from build123d import *

# Parameters (mm, degrees)
F0_W      = 16.5
F0_H      = 32.5
F1_DEPTH  = 14
F3_W      = 16.5
F3_H      = 17
F4_DEPTH  = 10
F5_W      = 4
F5_H      = 17
F6_DEPTH  = 14.001
F7_W      = 8.5
F7_H      = 4.5
F8_DEPTH  = 14.001
F9_R      = 2.85
F10_DEPTH = 3
F11_R     = 1
F12_DEPTH = 10


with BuildPart() as f1:
    # F0 (on Top) → F1 (new body)
    with BuildSketch(Plane.XY):
        Rectangle(F0_W, F0_H)
    extrude(amount=F1_DEPTH)

    # F3 (on face) → F4 (cut)
    with BuildSketch(Plane.XY.offset(14)):
        with Locations((0, 3.75)):
            Rectangle(F3_W, F3_H)
    extrude(amount=-F4_DEPTH, mode=Mode.SUBTRACT)

    # F5 (on face) → F6 (cut, through all)
    with BuildSketch(Plane(origin=(0, 0, 0), x_dir=(1, 0, 0), z_dir=(0, 0, -1))):
        with Locations((-6.25, -3.75)):
            Rectangle(F5_W, F5_H)
        with Locations((6.25, -3.75)):
            Rectangle(F5_W, F5_H)
    extrude(amount=-F6_DEPTH, mode=Mode.SUBTRACT)

    # F7 (on face) → F8 (cut, through all)
    with BuildSketch(Plane.XY.offset(14)):
        with Locations((0, -10.5)):
            Rectangle(F7_W, F7_H)
    extrude(amount=-F8_DEPTH, mode=Mode.SUBTRACT)

    # F9 (on face) → F10 (cut)
    with BuildSketch(Plane.XZ.offset(16.25)):
        with Locations((0, 7)):
            Circle(F9_R)
    extrude(amount=-F10_DEPTH, mode=Mode.SUBTRACT)

    # F11 (on face) → F12 (cut)
    with BuildSketch(Plane.XZ.offset(13.25)):
        with Locations((0, 7)):
            Circle(F11_R)
    extrude(amount=-F12_DEPTH, mode=Mode.SUBTRACT)


solid = f1.part
Design review of the part built by this model. Coordinates are the model's own, in mm. A direction names the side the tool comes from. Round coordinates to 2 decimals unless told otherwise and drop trailing zeros. Loops run counter-clockwise (first coordinate to the right, second up) from the corner with the lowest first, then second, coordinate; pieces in that order, holes last. Notation, with made-up numbers: (5.5, -15.5) - (35.5, -15.5) arc R18 cw to (35.5, 16.5) - close; hole circle Ø5 at (69, 32). An arc over 180 degrees is marked (long way). One line per item, written item: value. Start each with the question number.
1) Consider section A-A on z = 11.25. Give the boundary of the cut face in (x, y).
2) For faces 1 (the flat face through (0, 4, 4)), 2 (the cylindrical face through (-0.371, -14.771, 9.826)), 3 (the flat face through (-4.25, 4, 2)), 4 (the flat face through (-4.25, -11, 7)), list the 3-axis set-ups (+Z, -Z, +X, -X, +Y, -Y) from which the entire face can be reached by the end or side of a thin tool; tool diameter is ignored.
3) Insertion check: pin 1 Ø4 at (x, y) = (2, 1) entering from +Z; pin 2 Ø1.5 at (y, z) = (0.5, 2.5) entering from -X; pin 3 Ø3 at (y, z) = (3.5, 2.5) entering from +X; pin 4 Ø1.5 at (x, y) = (-6.5, 3.5) entering from -Z. Each pin has a flat end and moves straight along its axis. Give the tip position at first contact, or say it passes through.
4) Consider section C-C on y = -11. Give the boundary of the cut face in (x, z), then the cut area to 3 significant figures.
5) Draft analysis for pull direction X (two halves, no side actions). For faces 5 (the flat face through (4.25, 4, 2)), 6 (the flat face through (0, 0, 0)), 7 (the flat face through (4.25, -11, 7)), state which applies: +X half, -X half, draft (parallel to the pull), parting line (faces both ways), or undercut.
6) Consider section B-B on x = 0. Give the boundary of the cut face in (y, z).
7) To check wall thickness, follow L1, parallel to Y at x = -1.5, z = 8.5; L2, parallel to Y at x = -2.75, z = 13.25; L3, parallel to Z at x = 0, y = -13.1. State the ranges of each line that lie inside material, in increasing order. Write a range as from..to.
8) Consider section D-D on z = 1. Give the boundary of the cut face in (x, y), then the cut area to 3 significant figures.
Reported:
1. outline: (-8.25, -16.25) - (8.25, -16.25) - (8.25, -4.75) - (-8.25, -4.75) - close; (-8.25, 12.25) - (8.25, 12.25) - (8.25, 16.25) - (-8.25, 16.25) - close; hole (-4.25, -12.75) - (4.25, -12.75) - (4.25, -8.25) - (-4.25, -8.25) - close
2. face 1: +Z, +X, -X
2. face 2: -Y
2. face 3: +Z, -Z, -X
2. face 4: +Z, -Z
3. pin 1: stops at z = 4
3. pin 2: stops at x = -4.25
3. pin 3: stops at x = 4.25
3. pin 4: passes through
4. outline: (-8.25, 0) - (-4.25, 0) - (-4.25, 14) - (-8.25, 14) - close; (4.25, 0) - (8.25, 0) - (8.25, 14) - (4.25, 14) - close
4. area: 112 mm^2
5. face 5: +X half
5. face 6: draft
5. face 7: undercut
6. outline: (-16.25, 0) - (-12.75, 0) - (-12.75, 6) - (-13.25, 6) - (-13.25, 4.15) - (-16.25, 4.15) - close; (-16.25, 9.85) - (-13.25, 9.85) - (-13.25, 8) - (-12.75, 8) - (-12.75, 14) - (-16.25, 14) - close; (-8.25, 0) - (16.25, 0) - (16.25, 14) - (12.25, 14) - (12.25, 4) - (-4.75, 4) - (-4.75, 6) - (-8.25, 6) - close; (-8.25, 8) - (-4.75, 8) - (-4.75, 14) - (-8.25, 14) - close
7. L1: y = -13.25..-12.75, -8.25..-4.75, 12.25..16.25
7. L2: y = -16.25..-12.75, -8.25..-4.75, 12.25..16.25
7. L3: z = 0..6, 8..14
8. outline: (-8.25, -16.25) - (8.25, -16.25) - (8.25, -4.75) - (4.25, -4.75) - (4.25, 12.25) - (8.25, 12.25) - (8.25, 16.25) - (-8.25, 16.25) - (-8.25, 12.25) - (-4.25, 12.25) - (-4.25, -4.75) - (-8.25, -4.75) - close; hole (-4.25, -12.75) - (4.25, -12.75) - (4.25, -8.25) - (-4.25, -8.25) - close
8. area: 362 mm^2
